from build123d import *

# Parameters (mm, degrees)
F0_R     = 18
F0_R_2   = 15
F1_DEPTH = 30
F0_R_3   = 45
F2_DEPTH = 3
F3_R     = 1
F4_DEPTH = 32.8
F5_DEPTH = 25


with BuildPart() as f1:
    # F0 (on Top) → F1 (new body)
    with BuildSketch(Plane.XY):
        Circle(F0_R)
        Circle(F0_R_2, mode=Mode.SUBTRACT)
    extrude(amount=F1_DEPTH)

    # F0 (on Top) → F2 (join)
    with BuildSketch(Plane.XY):
        Circle(F0_R_3)
        Circle(F0_R, mode=Mode.SUBTRACT)
    extrude(amount=F2_DEPTH)

    # F3 (on face) → F4 (cut)
    with BuildSketch(Plane.XY.offset(3)):
        with Locations((3.380115, 18.891523)):
            Circle(F3_R)
    extrude(amount=-F4_DEPTH, mode=Mode.SUBTRACT)

    # F3 (on face) → F5 (cut)
    with BuildSketch(Plane.XY.offset(3)):
        with Locations((3.380115, 18.891523)):
            Circle(F3_R)
        with Locations((11.080593, 41.789821)):
            Circle(F3_R)
    extrude(amount=-F5_DEPTH, mode=Mode.SUBTRACT)


solid = f1.part
Could you check a few things on this model? Use its own coordinates, in mm. A direction names the side the tool comes from. Give positions to 0.01 mm unless a question says otherwise; leave off trailing zeros. Order: outer loops, then holes, each group sorted by start corner. A loop starts at its lowest first (then second) coordinate and runs counter-clockwise, first axis right, second up. Notation, with made-up numbers: (-34.5, 2) - (-26.5, 2) arc R14 cw to (-26.5, 13) - close; hole circle Ø5 at (7, 68.5). An arc over 180 degrees is marked (long way). Return JSON: item names as keys, results as strings. Group by question number.
Q1. Thinking about a two-plate mould opening in Y: for faces 3 (the face through (-14.985, 0.66, 14.79)), 4 (the face through (-2.343, 17.847, 16.311)), 5 (the face through (10.864, 40.814, 1.521)), 6 (the face through (-11, 11, 0)), which applies, pulls with the +Y half, pulls with the -Y half, needs draft (parallel to the pull), parting line crosses it, or undercut?
Q2. Which directions (+Z, -Z, +X, -X, +Y, -Y) give clear straight access to the entire face, cutting with the end or side of a thin tool? Please do faces 1 (the face through (19, 1, 3)), 2 (the face through (-4, 15, 30)).
Q3. Suppose I cut it at D-D, the plane y = -34. Please give me the cut outline in (x, z), and give its area (3 significant figures).
Q4. Suppose I cut it at A-A, the plane x = 0. Please give me the cut outline in (y, z).
Q5. Will these pins go through, and if not, where does the flat tip stop? pin 1 Ø10 at (x, z) = (19, 8.5) entering from +Y; pin 2 Ø8 at (x, z) = (-6.5, 23.5) entering from +Y.
Q6. Suppose I cut it at C-C, the plane z = 15.5. Please give me the cut outline in (x, y).
Q7. Please list where these lines run through material, in increasing order: line 1 along Y through (x, z) = (0, 14); line 2 along Z through (x, y) = (-26, -24.5); line 3 along X through (y, z) = (1.5, 24). Write a range as [from, to].
Resolved:
{
 "1": {"face 3": "undercut", "face 4": "parting line crosses it", "face 5": "undercut", "face 6": "needs draft"},
 "2": {"face 1": "+Z", "face 2": "+Z, +X, -X, +Y, -Y"},
 "3": {"outline": "(-29.48, 0) - (29.48, 0) - (29.48, 3) - (-29.48, 3) - close", "area": "177 mm2"},
 "4": {"outline": "(-45, 0) - (-15, 0) - (-15, 30) - (-18, 30) - (-18, 3) - (-45, 3) - close; (15, 0) - (45, 0) - (45, 3) - (18, 3) - (18, 30) - (15, 30) - close"},
 "5": {"pin 1": "stops at y = 11.31", "pin 2": "stops at y = 17.83"},
 "6": {"outline": "circle Ø36 at (0, 0); hole circle Ø30 at (0, 0)"},
 "7": {"line 1": "y = [-18, -15], [15, 18]", "line 2": "z = [0, 3]", "line 3": "x = [-17.94, -14.92], [14.92, 17.94]"}
}
